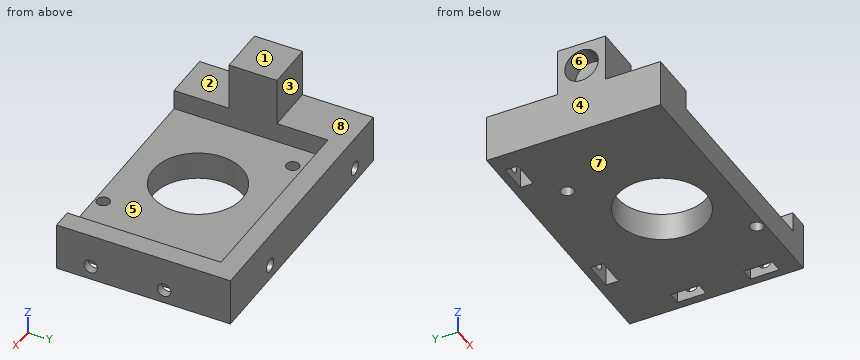
```python
from build123d import *

# Parameters (mm, degrees)
SKETCH_W        = 67.5
SKETCH_H        = 43.5
SKETCH_R        = 11.2
SKETCH_R_2      = 1.6
SKETCH_W_2      = 7.2
SKETCH_H_2      = 3.2
SKETCH_W_3      = 3.2
SKETCH_H_3      = 7.2
PAD_DEPTH       = 7
PAD001_DEPTH    = 5
SKETCH002_W     = 12
SKETCH002_H     = 12
PAD002_DEPTH    = 12
SKETCH003_R     = 4.2
POCKET_DEPTH    = 5
SKETCH004_R     = 1.7
POCKET001_DEPTH = 5
SKETCH005_R     = 1.7
POCKET002_DEPTH = 5


with BuildPart() as part:
    # Sketch → Pad (new body)
    with BuildSketch(Plane.XY):
        Rectangle(SKETCH_W, SKETCH_H)
        with Locations((0, -4.25)):
            Circle(SKETCH_R, mode=Mode.SUBTRACT)
        with Locations((-15.5, 11.25)):
            Circle(SKETCH_R_2, mode=Mode.SUBTRACT)
        with Locations((15.5, -19.75)):
            Circle(SKETCH_R_2, mode=Mode.SUBTRACT)
        with Locations((15.15, 18.15)):
            Rectangle(SKETCH_W_2, SKETCH_H_2, mode=Mode.SUBTRACT)
        with Locations((-25.15, 18.15)):
            Rectangle(SKETCH_W_2, SKETCH_H_2, mode=Mode.SUBTRACT)
        with Locations((30.15, 5.15)):
            Rectangle(SKETCH_W_3, SKETCH_H_3, mode=Mode.SUBTRACT)
        with Locations((30.15, -13.15)):
            Rectangle(SKETCH_W_3, SKETCH_H_3, mode=Mode.SUBTRACT)
    extrude(amount=PAD_DEPTH)

    # Sketch001 → Pad001 (new body)
    with BuildSketch(Plane.XY.offset(7)):
        Polygon((28.75, -21.75), (33.75, -21.75), (33.75, 21.75), (-33.75, 21.75), (-33.75, -21.75), (-21.75, -21.75), (-21.75, 16.75), (28.75, 16.75), align=None)
    extrude(amount=PAD001_DEPTH)

    # Sketch002 → Pad002 (new body)
    with BuildSketch(Plane.XY.offset(12)):
        with Locations((-27.75, -2)):
            Rectangle(SKETCH002_W, SKETCH002_H)
    extrude(amount=PAD002_DEPTH)

    # Sketch003 → Pocket (cut)
    with BuildSketch(Plane(origin=(-33.75, 0, 0), x_dir=(0, -1, 0), z_dir=(-1, 0, 0))):
        with Locations((2, 18)):
            Circle(SKETCH003_R)
    extrude(amount=-POCKET_DEPTH, mode=Mode.SUBTRACT)

    # Sketch004 → Pocket001 (cut)
    with BuildSketch(Plane(origin=(0, 21.75, 0), x_dir=(-1, 0, 0), z_dir=(0, 1, 0))):
        with Locations((25, 3.75)):
            Circle(SKETCH004_R)
        with Locations((-15, 3.75)):
            Circle(SKETCH004_R)
    extrude(amount=-POCKET001_DEPTH, mode=Mode.SUBTRACT)

    # Sketch005 → Pocket002 (cut)
    with BuildSketch(Plane.YZ.offset(33.75)):
        with Locations((5.15, 3.5)):
            Circle(SKETCH005_R)
        with Locations((-13.25, 3.5)):
            Circle(SKETCH005_R)
    extrude(amount=-POCKET002_DEPTH, mode=Mode.SUBTRACT)


solid = part.part
```
Part model, mm, in its own coordinate system. Face numbers are marked on the shaded views. A direction names the side the tool comes from. Round coordinates to 2 decimals unless told otherwise and drop trailing zeros. Loops run counter-clockwise (first coordinate to the right, second up) from the corner with the lowest first, then second, coordinate; pieces in that order, holes last.
Item 1: Cut at A-A, the plane x = 0. Give the cut face in (y, z).
Item 2: Cut at B-B, the plane z = 9. Give the cut face in (x, y), then the cut area to 3 significant figures.
Item 3: Cut at D-D, the plane y = -13.25. Give the cut face in (x, z).
Item 4: 3-axis set-ups, long thin cutter, end or side, ignore diameter. For the marked faces 1, 2, 3, 4 and 5: which of +Z, -Z, +X, -X, +Y, -Y reach the whole face in a straight line?
Item 5: Drill centre lines: line 1 (Z direction, x = 15, y = 21.1); line 2 (Y direction, x = 15.5, z = 5); line 3 (Y direction, x = 0, z = 3.25). Where is each one in solid material? Low to high.
Item 6: Drop flat-ended pins along their axis: P1, Ø1, axis at y = -16, z = 14, coming from the +X side; P2, Ø1.5, axis at x = 29.5, y = -12, coming from the -Z side; P3, Ø2, axis at y = -13.25, z = 3.5, coming from the +X side; P4, Ø22, axis at x = -4, y = 2.5, coming from the +Z side. Give the stop position or say it passes through.
Item 7: Mould opens along Z. For the marked faces 6, 7 and 8 say: +Z half, -Z half, draft (parallel to the pull), parting line (faces both ways), or undercut.
Item 8: Cut at C-C, the plane y = -1.5. Give the cut face in (x, z).
A:
1. outline: (-21.75, 0) - (-15.45, 0) - (-15.45, 7) - (-21.75, 7) - close; (6.95, 0) - (21.75, 0) - (21.75, 12) - (16.75, 12) - (16.75, 7) - (6.95, 7) - close
2. outline: (-33.75, -21.75) - (-21.75, -21.75) - (-21.75, 16.75) - (28.75, 16.75) - (28.75, -21.75) - (33.75, -21.75) - (33.75, 21.75) - (-33.75, 21.75) - close
2. area: 992 mm2
3. outline: (-33.75, 0) - (-6.67, 0) - (-6.67, 7) - (-21.75, 7) - (-21.75, 12) - (-33.75, 12) - close; (6.67, 0) - (28.55, 0) - (28.55, 7) - (6.67, 7) - close; (28.75, 7) - (31.75, 7) - (31.75, 5.2) - (33.75, 5.2) - (33.75, 12) - (28.75, 12) - close; (31.75, 0) - (33.75, 0) - (33.75, 1.8) - (31.75, 1.8) - close
4. face 1: +Z, +X, -X, +Y, -Y
4. face 2: +Z, +X, -X, -Y
4. face 3: +Z, +X, -X, +Y
4. face 4: +Z, -Z, -X, +Y, -Y
4. face 5: +Z, -Y
5. line 1: z = 0 to 2.05, 5.45 to 12
5. line 2: y = -21.75 to -21.35, -18.15 to 16.55
5. line 3: y = -21.75 to -15.45, 6.95 to 21.75
6. P1: passes through
6. P2: stops at z = 7
6. P3: stops at x = 28.55
6. P4: stops at z = 7
7. face 6: undercut
7. face 7: -Z half
7. face 8: +Z half
8. outline: (-33.75, 0) - (-10.86, 0) - (-10.86, 7) - (-21.75, 7) - (-21.75, 24) - (-33.75, 24) - (-33.75, 22.17) - (-28.75, 22.17) - (-28.75, 13.83) - (-33.75, 13.83) - close; (10.86, 0) - (33.75, 0) - (33.75, 12) - (28.75, 12) - (28.75, 7) - (10.86, 7) - close
